from build123d import *

# Parameters (mm, degrees)
F0_R     = 3.1623
F1_DEPTH = 10.033
F2_R     = 2.413
F3_DEPTH = 3.81
F4_R     = 0.381


with BuildPart() as f1:
    # F0 (on Front) → F1 (new body)
    with BuildSketch(Plane.XZ):
        Circle(F0_R)
    extrude(amount=-F1_DEPTH)

    # F2 (on Right) → F3 (cut, symmetric)
    with BuildSketch(Plane.YZ):
        with Locations((5.0165, 0)):
            Circle(F2_R)
    extrude(amount=F3_DEPTH, both=True, mode=Mode.SUBTRACT)

    # F4
    f4_edges = [f1.edges().sort_by_distance(p)[0] for p in [
        (-3.1623, 10.033, 0),
        (-3.1623, 0, 0),
    ]]
    fillet(f4_edges, radius=F4_R)


solid = f1.part
Can you work these out from the model? Positions are in its coordinate system, mm. Round coordinates to 2 decimals unless told otherwise and drop trailing zeros. Order: outer loops, then holes, each group sorted by start corner. A loop starts at its lowest first (then second) coordinate and runs counter-clockwise, first axis right, second up. Notation, with made-up numbers: (19, 35.5) - (61, 35.5) arc R26 cw to (61, 71.5) - close; hole circle Ø11 at (31, -15). An arc over 180 degrees is marked (long way). Answer in a Markdown table with one row per item.
(1) If we mould it in two halves opening along Y, with no side actions, what happens to faces 1 (the face through (0, 10.033, 0)), 2 (the face through (0, 0, 0)), 3 (the face through (0.04, 6.13, -2.14))? For each: released by +Y, released by -Y, zero draft, split by the parting line, or undercut.
From the geometry:
| item | result |
|---|---|
| face 1 | released by +Y |
| face 2 | released by -Y |
| face 3 | undercut |
(2) Suppose I cut it at A-A, the plane z = 0. Please give me the cut outline in (x, y), plus the area to 3 significant figures.
From the geometry:
| item | result |
|---|---|
| outline | (-3.16, 0.38) arc R0.38 ccw to (-2.78, 0) - (2.78, 0) arc R0.38 ccw to (3.16, 0.38) - (3.16, 2.6) - (-3.16, 2.6) - close; (-3.16, 7.43) - (3.16, 7.43) - (3.16, 9.65) arc R0.38 ccw to (2.78, 10.03) - (-2.78, 10.03) arc R0.38 ccw to (-3.16, 9.65) - close |
| area | 32.8 mm2 |
(3) Please list where these lines run through material, in increasing order: L1, parallel to Y at x = -1.5, z = 0; L2, parallel to Z at x = 1.5, y = 8.25; L3, parallel to Y at x = -1.5, z = 1.5. Write a range as from..to.
From the geometry:
| item | result |
|---|---|
| L1 | y = 0..2.6, 7.43..10.03 |
| L2 | z = -2.78..2.78 |
| L3 | y = 0..3.13, 6.91..10.03 |
(4) Suppose I cut it at C-C, the plane y = 6. Please give me the cut outline in (x, z), plus the area to 3 significant figures.
From the geometry:
| item | result |
|---|---|
| outline | (-2.27, -2.2) arc R3.16 ccw to (2.27, -2.2) - close; (-2.27, 2.2) - (2.27, 2.2) arc R3.16 ccw to start |
| area | 6.00 mm2 |
(5) Suppose I cut it at B-B, the plane x = 0. Please give me the cut outline in (y, z).
From the geometry:
| item | result |
|---|---|
| outline | (0, -2.78) arc R0.38 ccw to (0.38, -3.16) - (9.65, -3.16) arc R0.38 ccw to (10.03, -2.78) - (10.03, 2.78) arc R0.38 ccw to (9.65, 3.16) - (0.38, 3.16) arc R0.38 ccw to (0, 2.78) - close; hole circle Ø4.83 at (5.02, 0) |
(6) Suppose I cut it at D-D, the plane y = 4.75. Please give me the cut outline in (x, z), plus the area to 3 significant figures.
From the geometry:
| item | result |
|---|---|
| outline | (-2.06, -2.4) arc R3.16 ccw to (2.06, -2.4) - close; (-2.06, 2.4) - (2.06, 2.4) arc R3.16 ccw to start |
| area | 4.31 mm2 |
